For this review, take the finished solid that the model builds, in its own axes (mm). Round coordinates to 2 decimals unless told otherwise and drop trailing zeros. Write each loop counter-clockwise with the first axis right and the second up, starting at its lowest first coordinate (ties: lowest second). Pieces come first, ordered by that corner, then holes.
from build123d import *

# Parameters (mm, degrees)
SKETCH1_W           = 479
SKETCH1_H           = 711
BOSS_EXTRUDE1_DEPTH = 3.175
CUT_EXTRUDE1_DEPTH  = 429.696655574


with BuildPart() as part:
    # Sketch1 → Boss-Extrude1 (new, symmetric)
    with BuildSketch(Plane(origin=(0, 0, 0), x_dir=(1, 0, 0), z_dir=(0, 1, 0))):
        Rectangle(SKETCH1_W, SKETCH1_H)
    extrude(amount=BOSS_EXTRUDE1_DEPTH, both=True)

    # Sketch2 → Cut-Extrude1 (cut, through all)
    with BuildSketch(Plane(origin=(0, 3.175, 0), x_dir=(1, 0, 0), z_dir=(0, 1, 0))):
        Polygon((-239.5, 355.5), (-239.5, 255.5), (-233.15, 255.5), (-233.15, 349.15), (-139.5, 349.15), (-139.5, 355.5), align=None)
        Polygon((239.5, 355.5), (139.5, 355.5), (139.5, 349.15), (233.15, 349.15), (233.15, 255.5), (239.5, 255.5), align=None)
        Polygon((239.5, -355.5), (239.5, -255.5), (233.15, -255.5), (233.15, -349.15), (139.5, -349.15), (139.5, -355.5), align=None)
        Polygon((-239.5, -355.5), (-139.5, -355.5), (-139.5, -349.15), (-233.15, -349.15), (-233.15, -255.5), (-239.5, -255.5), align=None)
    extrude(amount=-CUT_EXTRUDE1_DEPTH, mode=Mode.SUBTRACT)


solid = part.part
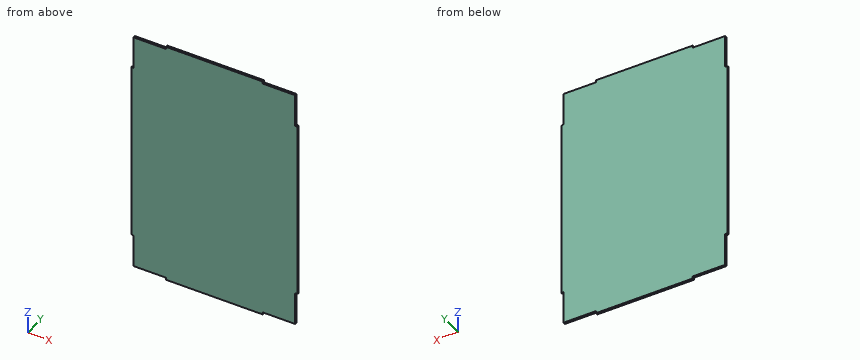
(1) For pin 1 Ø3 at (y, z) = (-1, 285) entering from +X; pin 2 Ø1.9 at (y, z) = (0.5, 353.5) entering from +X; pin 3 Ø1.9 at (y, z) = (-0.5, -353.5) entering from -X, all flat-tipped, find the tip position at first contact; note any pin that passes through.
Geometry check:
pin 1: stops at x = 233.15
pin 2: stops at x = 139.5
pin 3: stops at x = -139.5
(2) We need section B-B, the plane z = 266.5. Give the boundary of the cut face in (x, y) (3 decimals).
Geometry check:
outline: (-233.15, -3.175) - (233.15, -3.175) - (233.15, 3.175) - (-233.15, 3.175) - close
(3) For line 1 along X through (y, z) = (-1, -277); line 2 along Z through (x, y) = (-215.5, -1.5), list the stretches that pass through material, from the lowest coordinate up.
Geometry check:
line 1: x = -233.15 to 233.15
line 2: z = -349.15 to 349.15
(4) We need section A-A, the plane x = -179. Give the boundary of the cut face in (y, z) (3 decimals), and give its area (3 significant figures).
Geometry check:
outline: (-3.175, -349.15) - (3.175, -349.15) - (3.175, 349.15) - (-3.175, 349.15) - close
area: 4,430 mm2
